Design review of the part shown in the three views and the two pictorial views. Dimensions are in mm from the part's minimum x, y and z. Coordinates: 2 decimals unless noted, no trailing zeros. Write each loop counter-clockwise with the first axis right and the second up, starting at its lowest first coordinate (ties: lowest second). Pieces come first, ordered by that corner, then holes. Notation, with made-up numbers: (82.5, 55) -> (86.5, 55) arc R30 ccw to (86.5, 82) -> close; hole circle Ø1 at (-12, 4). An arc over 180 degrees is marked (long way). Answer in a Markdown table with one row per item. Add a question column.
Item 1: To check wall thickness, follow line 1 (Y direction, x = 3, z = 1.75); line 2 (Z direction, x = 2.85, y = 3.1); line 3 (Y direction, x = 0.4, z = 29). State the ranges of each line that lie inside material, in increasing order.
Item 2: Clearance check with flat-ended pins moving along their axes: P1, Ø1.7, axis at x = 3, y = 3, coming from the -Z side; P2, Ø0.8, axis at x = 3.5, y = 2.5, coming from the +Z side; P3, Ø1, axis at x = 1, z = 16.5, coming from the +Y side. State where each tip first meets the part, or that it passes through.
Item 3: Take a section at A-A, the plane x = 3. Write out the cut boundary in (y, z).
Item 4: Take a section at C-C, the plane z = 32.5. Write out the cut boundary in (x, y), and give its area (3 significant figures).
Item 5: Take a section at D-D, the plane z = 11. Write out the cut boundary in (x, y).
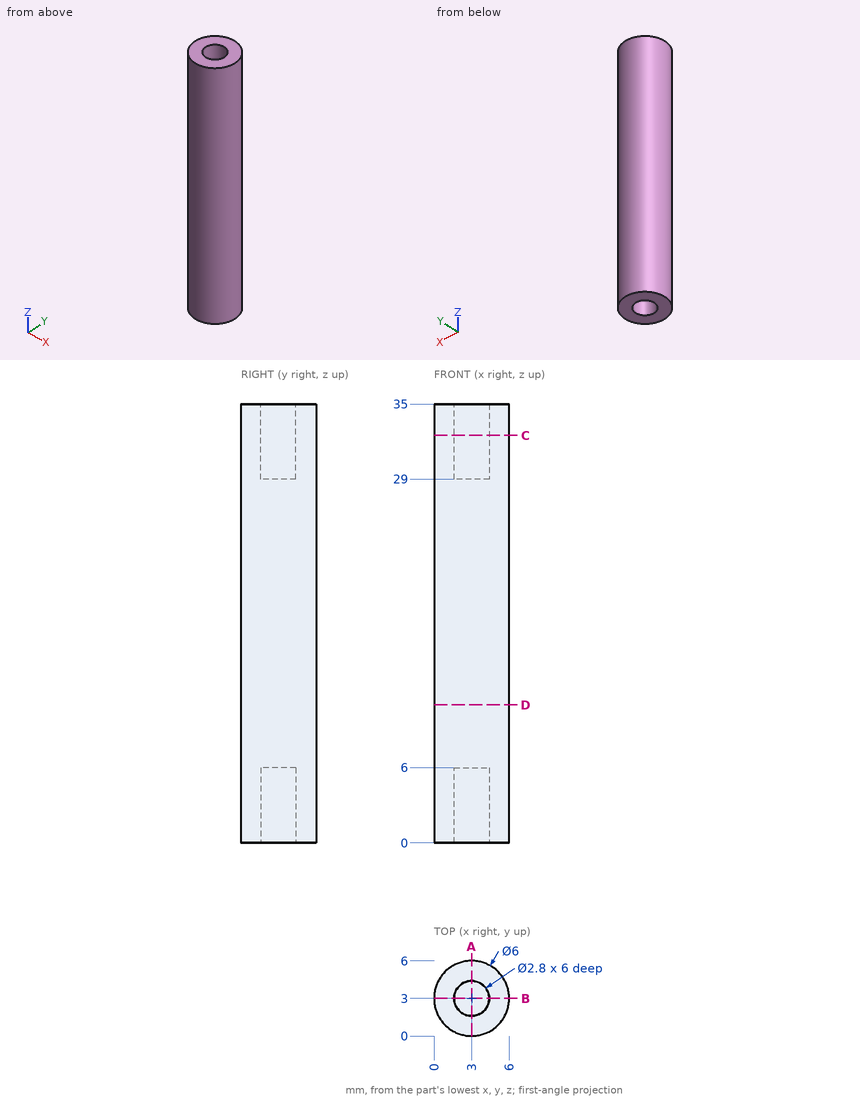
Answers:
| question | item | result |
|---|---|---|
| 1 | line 1 | y = 0 to 1.6, 4.4 to 6 |
| 1 | line 2 | z = 6 to 29 |
| 1 | line 3 | y = 1.5 to 4.5 |
| 2 | P1 | stops at z = 6 |
| 2 | P2 | stops at z = 29 |
| 2 | P3 | stops at y = 5.6 |
| 3 | outline | (0, 0) -> (1.6, 0) -> (1.6, 6) -> (4.4, 6) -> (4.4, 0) -> (6, 0) -> (6, 35) -> (4.4, 35) -> (4.4, 29) -> (1.6, 29) -> (1.6, 35) -> (0, 35) -> close |
| 4 | outline | circle Ø6 at (3, 3); hole circle Ø2.8 at (3, 3) |
| 4 | area | 22.1 mm^2 |
| 5 | outline | circle Ø6 at (3, 3) |
